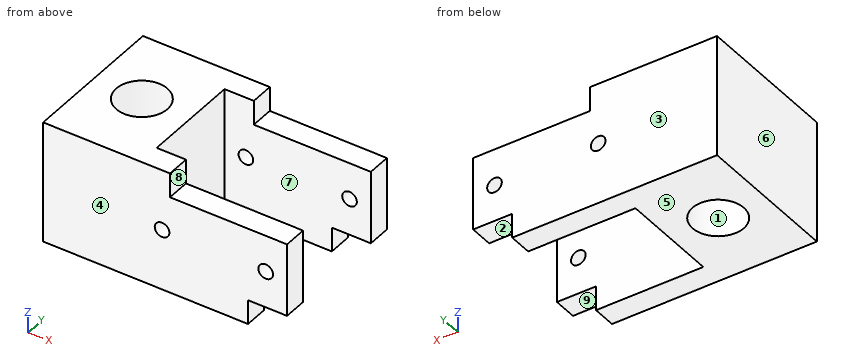
```python
from build123d import *

# Parameters (mm, degrees)
F0_W     = 25.4
F0_H     = 38.1
F1_DEPTH = 31.75
F2_W     = 6.096
F2_H     = 31.75
F3_DEPTH = 38.1
F4_R     = 6.6675
F5_DEPTH = 31.751
F6_R     = 1.905
F7_DEPTH = 38.101
F8_W     = 10.16
F8_H     = 6.35
F8_W_2   = 30.48
F9_DEPTH = 38.101


with BuildPart() as f1:
    # F0 (on Top) → F1 (new body)
    with BuildSketch(Plane.XY):
        Rectangle(F0_W, F0_H)
    extrude(amount=F1_DEPTH)

    # F2 (on face) → F3 (join)
    with BuildSketch(Plane.YZ.offset(12.7)):
        with Locations((-16.002, 15.875)):
            Rectangle(F2_W, F2_H)
        with Locations((16.002, 15.875)):
            Rectangle(F2_W, F2_H)
    extrude(amount=F3_DEPTH)

    # F4 (on face) → F5 (cut, through all)
    with BuildSketch(Plane.XY.offset(31.75)):
        Circle(F4_R)
    extrude(amount=-F5_DEPTH, mode=Mode.SUBTRACT)

    # F6 (on face) → F7 (cut, through all)
    with BuildSketch(Plane(origin=(0, 19.05, 0), x_dir=(-1, 0, 0), z_dir=(0, 1, 0))):
        with Locations((-45.24375, 15.875)):
            Circle(F6_R)
        with Locations((-18.25625, 15.875)):
            Circle(F6_R)
    extrude(amount=-F7_DEPTH, mode=Mode.SUBTRACT)

    # F8 (on face) → F9 (cut, through all)
    with BuildSketch(Plane.XZ.offset(19.05)):
        with Locations((45.72, 3.175)):
            Rectangle(F8_W, F8_H)
        with Locations((35.56, 28.575)):
            Rectangle(F8_W_2, F8_H)
    extrude(amount=-F9_DEPTH, mode=Mode.SUBTRACT)


solid = f1.part
```
Source: CAD feature listing. Evaluate the final solid. Frame: model axes, mm. Face numbers are marked on the shaded views. A direction names the side the tool comes from. Round coordinates to 2 decimals unless told otherwise and drop trailing zeros. Loops run counter-clockwise (first coordinate to the right, second up) from the corner with the lowest first, then second, coordinate; pieces in that order, holes last.
1. Mould query, pull axis Y, two halves, no side actions, for the marked faces 1, 2, 3 and 4. Classes: released by +Y, released by -Y, zero draft, split by the parting line, or undercut.
2. Contact query for flat-ended pins moving along their axis: pin 1 (13 mm diameter, centred on y = -6, z = 22.5, fed in from +X); pin 2 (1.8 mm diameter, centred on y = -15.5, z = 2, fed in from +X); pin 3 (1.8 mm diameter, centred on x = 32.5, y = -17.5, fed in from +Z). Output: stop coordinate, or through.
3. Section query D-D on z = 15. Give the number of separate pieces and of enclosed holes in the cut face, and give its area (3 significant figures).
4. Section query A-A on y = 0. Output: boundary loops of the cut face in (x, z).
5. Section query B-B on x = 33.5. Output: boundary loops of the cut face in (y, z).
6. Access query for the marked faces 5, 6, 7, 8 and 9. Directions: +Z, -Z, +X, -X, +Y, -Y. A direction counts if a zero-diameter tool reaches every point of the face in a straight line with its end or side. Return the directions, or none.
7. Ray query, L1, parallel to Y at x = 24.5, z = 4; L2, parallel to X at y = -5, z = 5.5; L3, parallel to X at y = -1.5, z = 7. Return the intervals inside material, ascending.
Answers below:
1. face 1: undercut
1. face 2: zero draft
1. face 3: released by +Y
1. face 4: released by -Y
2. pin 1: stops at x = 12.7
2. pin 2: stops at x = 40.64
2. pin 3: stops at z = 25.4
3. separate pieces: 5
3. enclosed holes: 1
3. area: 1,210 mm2
4. outline: (-12.7, 0) - (-6.67, 0) - (-6.67, 31.75) - (-12.7, 31.75) - close; (6.67, 0) - (12.7, 0) - (12.7, 31.75) - (6.67, 31.75) - close
5. outline: (-19.05, 0) - (-12.95, 0) - (-12.95, 25.4) - (-19.05, 25.4) - close; (12.95, 0) - (19.05, 0) - (19.05, 25.4) - (12.95, 25.4) - close
6. face 5: -Z, +X, -X, +Y, -Y
6. face 6: +Z, -Z, -X, +Y, -Y
6. face 7: +Z, -Z, +X
6. face 8: +Z, +X, +Y, -Y
6. face 9: -Z, +X, +Y, -Y
7. L1: y = -19.05 to -12.95, 12.95 to 19.05
7. L2: x = -12.7 to -4.41, 4.41 to 12.7
7. L3: x = -12.7 to -6.5, 6.5 to 12.7
